```python
from build123d import *

# Parameters (mm, degrees)
BOSS_EXTRUDE1_DEPTH            = 9.525
SKETCH2_W                      = 76.2
SKETCH2_H                      = 20.32
CUT_EXTRUDE1_DEPTH             = 12.7
SKETCH3_W                      = 19.05
SKETCH3_H                      = 101.6
CUT_EXTRUDE2_DEPTH             = 6.35
F_5_16_0_3125_DIAMETER_HOLE1_D = 7.9375
F_8_32_TAPPED_HOLE1_D          = 3.4544


with BuildPart() as part:
    # Sketch1 → Boss-Extrude1 (new, symmetric)
    with BuildSketch(Plane(origin=(0, 0, 0), x_dir=(1, 0, 0), z_dir=(0, 1, 0))):
        Polygon((-60.96, 22.225), (-60.96, -22.225), (-15.24, -50.8), (15.24, -50.8), (15.24, 50.8), (-15.24, 50.8), align=None)
    extrude(amount=BOSS_EXTRUDE1_DEPTH, both=True)

    # Sketch2 → Cut-Extrude1 (cut)
    with BuildSketch(Plane.XZ.offset(9.525)):
        with Locations((-22.86, 0)):
            Rectangle(SKETCH2_W, SKETCH2_H)
    extrude(amount=-CUT_EXTRUDE1_DEPTH, mode=Mode.SUBTRACT)

    # Sketch3 → Cut-Extrude2 (cut)
    with BuildSketch(Plane(origin=(0, 9.525, 0), x_dir=(1, 0, 0), z_dir=(0, 1, 0))):
        with Locations((5.715, 0)):
            Rectangle(SKETCH3_W, SKETCH3_H)
    extrude(amount=-CUT_EXTRUDE2_DEPTH, mode=Mode.SUBTRACT)

    # 5/16 (0.3125) Diameter Hole1 (through all)
    with Locations(Plane(origin=(0, 9.525, 0), x_dir=(1, 0, 0), z_dir=(0, 1, 0))):
        with Locations((-51.435, 0), (-32.385, 0), (-16.8275, 0)):
            Hole(F_5_16_0_3125_DIAMETER_HOLE1_D / 2)

    # #8-32 Tapped Hole1 (through all)
    with Locations(Plane(origin=(0, -9.525, 0), x_dir=(-1, 0, 0), z_dir=(0, -1, 0))):
        with Locations((-5.715, -25.4), (-5.715, 25.4)):
            Hole(F_8_32_TAPPED_HOLE1_D / 2)


solid = part.part
```
The model under review builds one solid part; all positions refer to its coordinate system, in mm. A direction names the side the tool comes from. Round coordinates to 2 decimals unless told otherwise and drop trailing zeros. Write each loop counter-clockwise with the first axis right and the second up, starting at its lowest first coordinate (ties: lowest second). Pieces come first, ordered by that corner, then holes.
(1) We need section D-D on z = -25.4. Give the boundary of the cut face in (x, y) (3 decimals).
(2) Insertion check: pin 1 (8 mm diameter, centred on x = -22, y = 0.5, fed in from +Z) (3 decimals); pin 2 (2 mm diameter, centred on x = -49, y = -7.5, fed in from +Z) (3 decimals); pin 3 (3 mm diameter, centred on y = 6, z = 36.5, fed in from +X). Each pin has a flat end and moves straight along its axis. Give the tip position at first contact, or say it passes through.
(3) We need section B-B on z = 0. Give the boundary of the cut face in (x, y) (3 decimals), and give its area (3 significant figures).
(4) We need section A-A on y = -3. Give the boundary of the cut face in (x, z) (3 decimals), and give its area (3 significant figures).
(5) Wall thickness on L1, parallel to Z at x = -8, y = -5.5; L2, parallel to Y at x = 10.5, z = -39 (3 decimals); L3, parallel to Z at x = -34, y = -5.5 (3 decimals): over which ranges is each line inside the solid? List them lowest first.
(6) We need section C-C on x = 10.5. Give the boundary of the cut face in (y, z) (3 decimals), and give its area (3 significant figures).
(7) Mouldability with a two-part tool opening along Z and no side actions: class faces 4 (the flat face through (-23, -3, -10.16)), 5 (the flat face through (0, -2, 50.8)), 6 (the flat face through (-3.81, 6, 1)) as +Z half, -Z half, draft (parallel to the pull), parting line (faces both ways), or undercut.
(8) Machinability: for faces 1 (the flat face through (6, 3.175, -31)), 2 (the flat face through (-33, 3.175, 5)), 3 (the flat face through (-38.42, 0.133, 36.312)), which of the approach directions +Z, -Z, +X, -X, +Y, -Y give a long, thin tool a straight path to every point of the face, cutting with its end or side? Answer none if there is none.
Findings below:
1. outline: (-55.88, -9.525) - (3.988, -9.525) - (3.988, 3.175) - (-3.81, 3.175) - (-3.81, 9.525) - (-55.88, 9.525) - close; (7.442, -9.525) - (15.24, -9.525) - (15.24, 3.175) - (7.442, 3.175) - close
2. pin 1: stops at z = 49.075
2. pin 2: stops at z = 30.325
2. pin 3: stops at x = -3.81
3. outline: (-60.96, 3.175) - (-55.404, 3.175) - (-55.404, 9.525) - (-60.96, 9.525) - close; (-47.466, 3.175) - (-36.354, 3.175) - (-36.354, 9.525) - (-47.466, 9.525) - close; (-28.416, 3.175) - (-20.796, 3.175) - (-20.796, 9.525) - (-28.416, 9.525) - close; (-12.859, 3.175) - (-3.81, 3.175) - (-3.81, 9.525) - (-12.859, 9.525) - close
3. area: 212 mm2
4. outline: (-60.96, -22.225) - (-15.24, -50.8) - (15.24, -50.8) - (15.24, -10.16) - (-60.96, -10.16) - close; (-60.96, 10.16) - (15.24, 10.16) - (15.24, 50.8) - (-15.24, 50.8) - (-60.96, 22.225) - close; hole circle Ø3.454 at (5.715, -25.4); hole circle Ø3.454 at (5.715, 25.4)
4. area: 4,870 mm2
5. L1: z = -50.8 to -10.16, 10.16 to 50.8
5. L2: y = -9.525 to 3.175
5. L3: z = -39.075 to -10.16, 10.16 to 39.075
6. outline: (-9.525, -50.8) - (3.175, -50.8) - (3.175, -10.16) - (-9.525, -10.16) - close; (-9.525, 10.16) - (3.175, 10.16) - (3.175, 50.8) - (-9.525, 50.8) - close
6. area: 1,030 mm2
7. face 4: undercut
7. face 5: +Z half
7. face 6: draft
8. face 1: +Z, -Z, +X, +Y
8. face 2: +X, -X, -Y
8. face 3: +Z, -X, +Y, -Y
